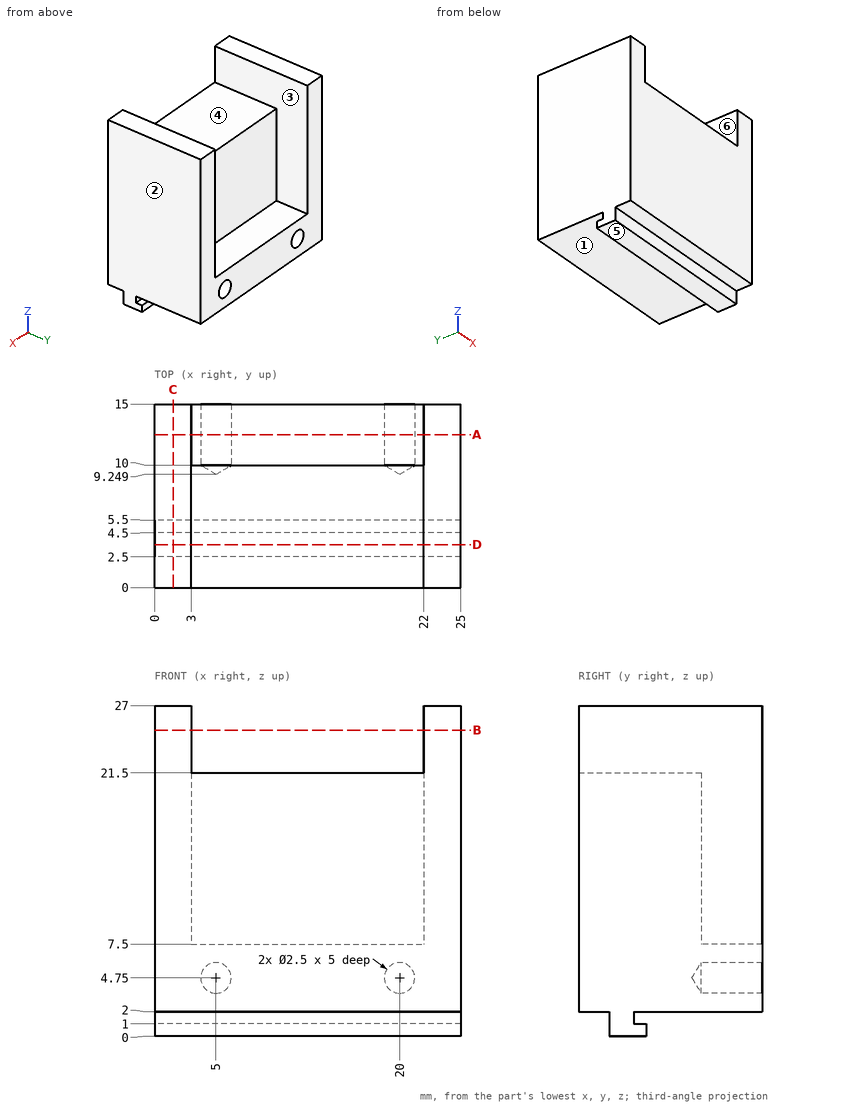
Check sheet for the drawn part. Datum: minimum x, y, z corner. Units: mm. A direction names the side the tool comes from. Give positions to 0.01 mm unless a question says otherwise; leave off trailing zeros. Loops run counter-clockwise (first coordinate to the right, second up) from the corner with the lowest first, then second, coordinate; pieces in that order, holes last.
1) Sectioned sample at D-D, the plane y = 3.5. Enter the section's corners in (x, z), then the cut area to 4 significant figures.
2) Sectioned sample at C-C, the plane x = 1.5. Enter the section's corners in (y, z), then the cut area to 3 significant figures.
3) Thickness scan on line 1 along X through (y, z) = (11.35, 4.75); line 2 along Z through (x, y) = (5, 13.7); line 3 along X through (y, z) = (10.5, 16.5). Record the ranges inside material, lowest first.
4) Set-up check for the marked faces 4, 5 and 6: record each of +Z, -Z, +X, -X, +Y, -Y from which the full face is reachable in a straight line by a thin tool's end or side.
5) Draft check along X on the marked faces 1, 2 and 3. Enter one of: pulls with the +X half, pulls with the -X half, needs draft (parallel to the pull), parting line crosses it, or undercut.
6) Depth check by flat-ended pin: pin 1 Ø0.8 at (x, z) = (6.5, 1.5) entering from +Y; pin 2 Ø2 at (x, z) = (5, 4.75) entering from +Y; pin 3 Ø2.5 at (x, y) = (11, 13.5) entering from +Z. Enter the tip coordinate at first touch or a pass-through.
7) Sectioned sample at A-A, the plane y = 12.5. Enter the section's corners in (x, z), then the cut area to 3 significant figures.
8) Sectioned sample at B-B, the plane z = 25. Enter the section's corners in (x, y), then the cut area to 3 significant figures.
Answers:
1. outline: (0, 0) - (25, 0) - (25, 27) - (22, 27) - (22, 21.5) - (3, 21.5) - (3, 27) - (0, 27) - close
1. area: 570.5 mm2
2. outline: (0, 2) - (2.5, 2) - (2.5, 0) - (5.5, 0) - (5.5, 1) - (4.5, 1) - (4.5, 2) - (15, 2) - (15, 27) - (0, 27) - close
2. area: 380 mm2
3. line 1: x = 0 to 3.75, 6.25 to 18.75, 21.25 to 25
3. line 2: z = 2 to 3.5, 6 to 7.5
3. line 3: x = 0 to 3, 22 to 25
4. face 4: +Z, +Y, -Y
4. face 5: -Z, +X, -X, +Y, -Y
4. face 6: +Z, +Y
5. face 1: needs draft
5. face 2: pulls with the +X half
5. face 3: undercut
6. pin 1: stops at y = 4.5
6. pin 2: stops at y = 9.85
6. pin 3: stops at z = 7.5
7. outline: (0, 2) - (25, 2) - (25, 27) - (22, 27) - (22, 7.5) - (3, 7.5) - (3, 27) - (0, 27) - close; hole circle Ø2.5 at (5, 4.75); hole circle Ø2.5 at (20, 4.75)
7. area: 245 mm2
8. outline: (0, 0) - (3, 0) - (3, 15) - (0, 15) - close; (22, 0) - (25, 0) - (25, 15) - (22, 15) - close
8. area: 90.0 mm2
